Autodesk Fusion 360 part; units mm, degrees
sketch "Boceto1" plane through (0, 0, 0) normal (0, 0, 1) x (1, 0, 0)
  line L0 (0, 72) -> (28, 72)
  line L1 (28, 72) -> (28, 0)
  line L2 (28, 0) -> (0, 0)
  line L3 (0, 0) -> (0, 72)
  dimension "d1" = 72
  dimension "d2" = 28
extrude "Extruir1" add sketch "Boceto1" along normal blind 1 makes body 1
sketch "Boceto2" plane through (0, 0, 0) normal (1, 0, 0) x (0, 1, 0)
  line L0 (0, 1) -> (0, 20)
  line L1 (0, 20) -> (12, 20)
  line L2 (12, 20) -> (15, 17)
  line L3 (15, 17) -> (57, 17)
  line L4 (57, 17) -> (60, 20)
  line L5 (60, 20) -> (72, 20)
  line L6 (72, 20) -> (72, 1)
  line L7 (72, 1) -> (0, 1)
  line L8 (0, 1) -> (72, 1)
  dimension "d5" = 19
  dimension "d6" = 12
  dimension "d7" = 12
  dimension "d8" = 72
  dimension "d9" = 45
  dimension "d12" = 16
extrude "Extruir2" add sketch "Boceto2" along normal blind 28 bodies 1
shell "Vaciado1" thickness 1 removed faces 5 at (9.3333, 4, 20) at (9.3333, 13, 19) at (9.3333, 29, 17) at (9.3333, 58, 18) at (9.3333, 64, 20) on bodies 1
sketch "Boceto5" plane through (0, 0, 0) normal (0, 0, -1) x (1, 0, 0)
  line L0 (28, 0) -> (0, 0)
  line L1 (0, 0) -> (0, -72)
  line L2 (0, -72) -> (28, -72)
  line L3 (28, -72) -> (28, 0)
  line L4 (0, 0) -> (0, 1.4)
  line L5 (28, 0) -> (28, 1.4)
  arc A0 (28, 1.4) -> (0, 1.4) centre (14, -56.9438) ccw
  line L6 (0, 0) -> (28, 0)
  dimension "d28" = 1.4
  dimension "d29" = 1.4
  dimension "d30" = 60
extrude "Extruir3" add sketch "Boceto5" against normal blind 1 separate body contours L0 L4 L5 A0 L6 makes body 2
sketch "Boceto6" plane through (0, 0, 1) normal (0, 0, 1) x (-1, 0, 0)
  line L0 (-28, 0) -> (0, 0)
  line L1 (0, 0) -> (0, 1.4)
  arc A0 (0, 1.4) -> (-28, 1.4) centre (-14, -56.9438) ccw
  line L2 (-28, 1.4) -> (-28, 0)
  line L3 (-5, 1) -> (-23, 1)
  arc A1 (-5, 1) -> (-23, 1) centre (-14, -37.9744) ccw
  line L4 (0, 0) -> (-28, 0)
  dimension "d35" = 18
  dimension "d36" = 5
  dimension "d37" = 40
  dimension "d38" = 1
extrude "Extruir4" cut sketch "Boceto6" against normal blind 1 contours L3 A1 bodies 2
sketch "Boceto7" plane through (0, 0, 1) normal (0, 0, 1) x (-1, 0, 0)
  line L0 (-5, 1) -> (-23, 1)
  arc A0 (-5, 1) -> (-23, 1) centre (-14, -37.9744) ccw
  line L1 (-28, 0) -> (0, 0)
  line L2 (0, 0) -> (0, 1.4)
  arc A1 (0, 1.4) -> (-28, 1.4) centre (-14, -56.9438) ccw
  line L3 (-28, 1.4) -> (-28, 0)
  line L4 (-1, 0) -> (0, 0)
  line L5 (-4, 2.217) -> (-4, 0.4)
  line L6 (-4, 0.4) -> (-1, 0.4)
  line L7 (-1, 0.4) -> (-1, 0)
  arc A2 (0, 1.4) -> (-4, 2.217) centre (-14, -56.9438) ccw
  line L8 (-14, -72) -> (-14, 0) construction
  line L9 (-24, 0.4) -> (-27, 0.4)
  line L10 (-27, 0.4) -> (-27, 0)
  line L11 (-27, 0) -> (-28, 0)
  line L12 (-28, 0) -> (-28, 1.4)
  arc A3 (-24, 2.217) -> (-28, 1.4) centre (-14, -56.9438) ccw
  line L13 (-24, 2.217) -> (-24, 0.4)
  dimension "d39" = 0.4
  dimension "d40" = 1
  dimension "d41" = 4
  dimension "d42" = 60
extrude "Extruir5" add sketch "Boceto7" along normal blind 19 contours L1 A1 L3 L9 L10 L11 L12 A3 L13 | L1 L2 A1 L4 L5 L6 L7 A2 bodies 1 2
equation "d1 = internal_depth + 2 mm"
equation "d2 = internal_width + 2 mm"
equation "d5 = internal_height"
equation "d6 = ( internal_depth + 2 mm ) / 6"
equation "d7 = ( internal_depth + 2 mm ) / 6"
equation "d8 = internal_depth + 2 mm"
equation "d12 = internal_height - 3 mm"
equation "internal_depth = 70 mm"
equation "internal_width = 26 mm"
equation "internal_height = 19 mm"
equation "wall_width = 1 mm"
equation "d24 = wall_width"
equation "d35 = ( internal_width + 2 mm ) - 10 mm"
equation "d43 = internal_height"
Work out the finished part from the listing and answer in its coordinate system (mm). A direction names the side the tool comes from. Give positions to 0.01 mm unless a question says otherwise; leave off trailing zeros. Order: outer loops, then holes, each group sorted by start corner. A loop starts at its lowest first (then second) coordinate and runs counter-clockwise, first axis right, second up. Notation, with made-up numbers: M 71.5,-21 L 120.5,-21 A14 ccw 120.5,-6 Z; hole C -17,-21 d3. An arc over 180 degrees is marked long. Return JSON: item names as keys, results as strings.
1) Section C-C, the plane y = 59 is taken. Write down the section's boundary in (x, z), plus the area to 3 significant figures.
Resolved:
{"outline": "M 0,0 L 28,0 L 28,19 L 27,19 L 27,1 L 1,1 L 1,19 L 0,19 Z", "area": "64.0 mm^2"}
2) Straight lines are drawn through the part: line 1 along Y through (x, z) = (8, 14.75); line 2 along X through (y, z) = (64.5, 13); line 3 along Y through (x, z) = (1.75, 8). For each, find the intervals that lie inside material, in ascending order. Write a range as [from, to].
Resolved:
{"line 1": "[0, 1], [71, 72]", "line 2": "[0, 1], [27, 28]", "line 3": "[-1.79, -0.4], [0, 1], [71, 72]"}
3) Section D-D, the plane z = 3.75 is taken. Write down the section's boundary in (x, y).
Resolved:
{"outline": "M 0,-1.4 A60 ccw 4,-2.22 L 4,-0.4 L 1,-0.4 L 1,0 L 27,0 L 27,-0.4 L 24,-0.4 L 24,-2.22 A60 ccw 28,-1.4 L 28,72 L 0,72 Z; hole M 1,1 L 27,1 L 27,71 L 1,71 Z"}
4) Each of these flat-tipped pins is pushed along its axis until it touches: pin 1 (0.8 mm diameter, centred on x = 0.5, y = 33.5, fed in from +Z); pin 2 (1 mm diameter, centred on x = 8.5, y = 61, fed in from +Z); pin 3 (12 mm diameter, centred on x = 4.5, z = 15.5, fed in from -Y). Where does it stop, or does it pass through?
Resolved:
{"pin 1": "z = 17", "pin 2": "z = 1", "pin 3": "y = -2.22"}
5) For a pull along Y with two mould halves and no side action, classify faces 1 (the flat face through (27.5, 13.5, 18.5)), 2 (the flat face through (14, 71, 10)), 3 (the flat face through (14, 35, 0)), 4 (the cylindrical face through (13.02, -3.05, 0.32)) as +Y half, -Y half, draft (parallel to the pull), parting line (faces both ways), or undercut.
Resolved:
{"face 1": "undercut", "face 2": "undercut", "face 3": "draft", "face 4": "-Y half"}
6) A tool of negligible diameter and unlimited length cuts with its end or side. For faces 5 (the flat face through (0, 35, 10)), 6 (the flat face through (27.5, 58.5, 18.5)), 7 (the flat face through (14, 1, 10)), 8 (the flat face through (4, -1, 10)), from which of +Z, -Z, +X, -X, +Y, -Y can it reach the whole face along a straight path? Write none if from no direction.
Resolved:
{"face 5": "+Z, -Z, -X, +Y, -Y", "face 6": "+Z, +X, -X", "face 7": "+Z", "face 8": "+Z, -Y"}
7) Section A-A, the plane z = 17.75 is taken. Write down the section's boundary in (x, y).
Resolved:
{"outline": "M 0,-1.4 A60 ccw 4,-2.22 L 4,-0.4 L 1,-0.4 L 1,0 L 27,0 L 27,-0.4 L 24,-0.4 L 24,-2.22 A60 ccw 28,-1.4 L 28,14.25 L 27,14.25 L 27,1 L 1,1 L 1,14.25 L 0,14.25 Z; M 0,57.75 L 1,57.75 L 1,71 L 27,71 L 27,57.75 L 28,57.75 L 28,72 L 0,72 Z"}
8) Section B-B, the plane x = 21.5 is taken. Write down the section's boundary in (y, z).
Resolved:
{"outline": "M -2.59,0 L -1.32,0 L -1.32,1 L -2.59,1 Z; M -1,0 L 72,0 L 72,20 L 71,20 L 71,1 L 1,1 L 1,20 L 0,20 L 0,1 L -1,1 Z"}
